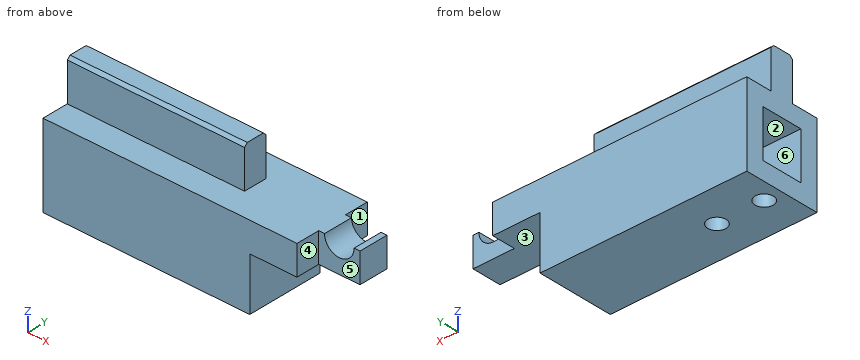
```python
from build123d import *

# Parameters (mm, degrees)
SKETCH_1_W                      = 25
SKETCH_1_H                      = 17
EXTRUDE_1_DEPTH                 = 50
SKETCH_2_W                      = 11
SKETCH_2_H                      = 6
CUT_EXTRUDE_1_DEPTH             = 50
SKETCH_3_W                      = 20
SKETCH_3_H                      = 11
CUT_EXTRUDE_2_DEPTH             = 50
SKETCH_4_W                      = 7
SKETCH_4_H                      = 6
CUT_EXTRUDE_3_DEPTH             = 50
SKETCH_5_W                      = 7
SKETCH_5_H                      = 9
CUT_EXTRUDE_4_DEPTH             = 50
SKETCH_6_R                      = 2.5
CUT_EXTRUDE_5_DEPTH             = 50
SKETCH_7_W                      = 14
SKETCH_7_H                      = 2
CUT_EXTRUDE_8_DEPTH             = 50
SKETCH_10_W                     = 4
SKETCH_10_H                     = 5
CUT_EXTRUDE_9_DEPTH             = 50
SKETCH_11_W                     = 8
SKETCH_11_H                     = 7
CUT_EXTRUDE_10_DEPTH            = 30
CUT_EXTRUDE_11_DEPTH            = 50
CUT_EXTRUDE_12_DEPTH            = 50
SKETCH_14_R                     = 1.55
CUT_EXTRUDE_13_DEPTH            = 5
SKIZZE1_W                       = 9
SKIZZE1_H                       = 13
SCHNITT_LINEAR_AUSTRAGEN1_DEPTH = 8


with BuildPart() as part:
    # 草图1 → 凸台-拉伸1 (new body)
    with BuildSketch(Plane(origin=(0, 0, 0), x_dir=(0, 0, -1), z_dir=(1, 0, 0))):
        with Locations((12.5, 8.5)):
            Rectangle(SKETCH_1_W, SKETCH_1_H)
    extrude(amount=EXTRUDE_1_DEPTH)

    # 草图2 → 切除-拉伸1 (cut)
    with BuildSketch(Plane.ZY):
        with Locations((-5.5, 14)):
            Rectangle(SKETCH_2_W, SKETCH_2_H)
        with Locations((-5.5, 3)):
            Rectangle(SKETCH_2_W, SKETCH_2_H)
    extrude(amount=-CUT_EXTRUDE_1_DEPTH, mode=Mode.SUBTRACT)

    # 草图3 → 切除-拉伸2 (cut)
    with BuildSketch(Plane(origin=(0, 11, 0), x_dir=(1, 0, 0), z_dir=(0, 1, 0))):
        with Locations((40, 5.5)):
            Rectangle(SKETCH_3_W, SKETCH_3_H)
    extrude(amount=-CUT_EXTRUDE_2_DEPTH, mode=Mode.SUBTRACT)

    # 草图4 → 切除-拉伸3 (cut)
    with BuildSketch(Plane(origin=(0, 0, -25), x_dir=(-1, 0, 0), z_dir=(0, 0, -1))):
        with Locations((-46.5, 14)):
            Rectangle(SKETCH_4_W, SKETCH_4_H)
        with Locations((-46.5, 3)):
            Rectangle(SKETCH_4_W, SKETCH_4_H)
    extrude(amount=-CUT_EXTRUDE_3_DEPTH, mode=Mode.SUBTRACT)

    # 草图5 → 切除-拉伸4 (cut)
    with BuildSketch(Plane(origin=(0, 11, 0), x_dir=(1, 0, 0), z_dir=(0, 1, 0))):
        with Locations((46.5, 20.5)):
            Rectangle(SKETCH_5_W, SKETCH_5_H)
    extrude(amount=-CUT_EXTRUDE_4_DEPTH, mode=Mode.SUBTRACT)

    # 草图6 → 切除-拉伸5 (cut)
    with BuildSketch(Plane(origin=(0, 11, 0), x_dir=(1, 0, 0), z_dir=(0, 1, 0))):
        with Locations((46.5, 11)):
            Circle(SKETCH_6_R)
    extrude(amount=-CUT_EXTRUDE_5_DEPTH, mode=Mode.SUBTRACT)

    # 草图7 → 切除-拉伸8 (cut)
    with BuildSketch(Plane.ZY):
        with Locations((-18, 16)):
            Rectangle(SKETCH_7_W, SKETCH_7_H)
        with Locations((-18, 1)):
            Rectangle(SKETCH_7_W, SKETCH_7_H)
    extrude(amount=-CUT_EXTRUDE_8_DEPTH, mode=Mode.SUBTRACT)

    # 草图10 → 切除-拉伸9 (cut)
    with BuildSketch(Plane.ZY):
        with Locations((-2, 8.5)):
            Rectangle(SKETCH_10_W, SKETCH_10_H)
    extrude(amount=-CUT_EXTRUDE_9_DEPTH, mode=Mode.SUBTRACT)

    # 草图11 → 切除-拉伸10 (cut)
    with BuildSketch(Plane.ZY):
        with Locations((-18, 8.5)):
            Rectangle(SKETCH_11_W, SKETCH_11_H)
    extrude(amount=-CUT_EXTRUDE_10_DEPTH, mode=Mode.SUBTRACT)

    # 草图12 → 切除-拉伸11 (cut)
    with BuildSketch(Plane.ZY):
        Polygon((-4, 11), (-4, 10), (-5, 11), align=None)
        Polygon((-4, 6), (-5, 6), (-4, 7), align=None)
    extrude(amount=-CUT_EXTRUDE_11_DEPTH, mode=Mode.SUBTRACT)

    # 草图13 → 切除-拉伸12 (cut)
    with BuildSketch(Plane.ZY):
        Polygon((-11, 11), (-11, 10.5), (-4.5, 10.5), (-5, 11), align=None)
        Polygon((-4.5, 6.5), (-5, 6), (-11, 6), (-11, 6.5), align=None)
    extrude(amount=-CUT_EXTRUDE_12_DEPTH, mode=Mode.SUBTRACT)

    # 草图14 → 切除-拉伸13 (cut)
    with BuildSketch(Plane(origin=(0, 0, -25), x_dir=(-1, 0, 0), z_dir=(0, 0, -1))):
        with Locations((-3, 8.5)):
            Circle(SKETCH_14_R)
        with Locations((-11, 8.5)):
            Circle(SKETCH_14_R)
    extrude(amount=-CUT_EXTRUDE_13_DEPTH, mode=Mode.SUBTRACT)

    # Skizze1 → Schnitt-Linear austragen1 (cut)
    with BuildSketch(Plane(origin=(43, 0, 0), x_dir=(0, 0, -1), z_dir=(1, 0, 0))):
        with Locations((20.5, 8.5)):
            Rectangle(SKIZZE1_W, SKIZZE1_H)
    extrude(amount=-SCHNITT_LINEAR_AUSTRAGEN1_DEPTH, mode=Mode.SUBTRACT)


solid = part.part
```
Can you work these out from the model? Positions are in its coordinate system, mm. Face numbers are marked on the shaded views. A direction names the side the tool comes from. Round coordinates to 2 decimals unless told otherwise and drop trailing zeros. Order: outer loops, then holes, each group sorted by start corner. A loop starts at its lowest first (then second) coordinate and runs counter-clockwise, first axis right, second up. Notation, with made-up numbers: (-8.5, -36.75) -> (50.5, -36.75) arc R18 ccw to (50.5, -13.75) -> close; hole circle Ø5 at (82, -2.75). An arc over 180 degrees is marked (long way). Return JSON: item names as keys, results as strings. Group by question number.
1. If we section it at D-D, the plane z = -20.75: Write out the boundary of the cut face in (x, y), then the cut area to 3 significant figures.
2. We'd pull the mould along Y, two halves only. Please class the marked faces 4, 5 and 6: released by +Y, released by -Y, zero draft, split by the parting line, or undercut.
3. If we section it at A-A, the plane y = 8.5: Write out the boundary of the cut face in (x, z), then the cut area to 3 significant figures.
4. I need wall thicknesses on line 1 (Z direction, x = 22, y = 5.5); line 2 (Y direction, x = 2, z = -17.5); line 3 (Y direction, x = 3, z = -22.9). Which ranges of each line are inside material? Lowest first, please. Write a range as [from, to].
5. If we section it at B-B, the plane z = -11.5: Write out the boundary of the cut face in (x, y), then the cut area to 3 significant figures.
6. Will these pins go through, and if not, where does the flat tip stop? pin 1 (4.5 mm diameter, centred on y = 11.5, z = -22.5, fed in from +X); pin 2 (2 mm diameter, centred on x = 8, y = 3.5, fed in from +Z); pin 3 (2 mm diameter, centred on y = 8.5, z = -16.5, fed in from -X).
7. If we section it at C-C, the plane x = 27.5: Write out the boundary of the cut face in (y, z).
8. Which directions (+Z, -Z, +X, -X, +Y, -Y) give clear straight access to the entire face, cutting with the end or side of a thin tool? Please do the marked faces 1, 2 and 3.
Output values:
{
 "1": {"outline": "(0, 2) -> (35, 2) -> (35, 15) -> (0, 15) -> (0, 12) -> (30, 12) -> (30, 5) -> (0, 5) -> close", "area": "245 mm²"},
 "2": {"face 4": "zero draft", "face 5": "released by -Y", "face 6": "undercut"},
 "3": {"outline": "(0, -25) -> (1.45, -25) -> (1.45, -22) -> (0, -22) -> close; (0, -14) -> (30, -14) -> (30, -22) -> (12.55, -22) -> (12.55, -25) -> (35, -25) -> (35, -16) -> (50, -16) -> (50, -11) -> (49, -11) arc R2.5 cw to (44, -11) -> (30, -11) -> (30, -4) -> (0, -4) -> close; (4.55, -25) -> (9.45, -25) -> (9.45, -22) -> (4.55, -22) -> close", "area": "507 mm²"},
 "4": {"line 1": "[-25, -22], [-14, -11]", "line 2": "[2, 5], [12, 15]", "line 3": "[2, 6.95], [10.05, 15]"},
 "5": {"outline": "(0, 2) -> (43, 2) -> (43, 6) -> (44.05, 6) -> (44.05, 11) -> (43, 11) -> (43, 15) -> (0, 15) -> close; (48.95, 6) -> (50, 6) -> (50, 11) -> (48.95, 11) -> close", "area": "570 mm²"},
 "6": {"pin 1": "x = 35", "pin 2": "z = -11", "pin 3": "x = 30"},
 "7": {"outline": "(2, -25) -> (15, -25) -> (15, -11) -> (10.5, -11) -> (10.5, -4.5) -> (10, -4) -> (7, -4) -> (6.5, -4.5) -> (6.5, -11) -> (2, -11) -> close; hole (5, -22) -> (12, -22) -> (12, -14) -> (5, -14) -> close"},
 "8": {"face 1": "+Z, -Z, +X, +Y", "face 2": "-X", "face 3": "-Z, +X, +Y, -Y"}
}
